The listing builds one solid part. Answer for the finished solid, in the listing's coordinates (mm). Face numbers are marked on the shaded views. A direction names the side the tool comes from. Round coordinates to 2 decimals unless told otherwise and drop trailing zeros. Write each loop counter-clockwise with the first axis right and the second up, starting at its lowest first coordinate (ties: lowest second). Pieces come first, ordered by that corner, then holes. Notation, with made-up numbers: (60.25, -40) - (118.25, -40) arc R27 cw to (118.25, -14) - close; hole circle Ø2 at (57, 41.5). An arc over 180 degrees is marked (long way). Return JSON: item names as keys, results as strings. Group by question number.
from build123d import *

# Parameters (mm, degrees)
SKETCH1_R           = 8.75
SKETCH1_R_2         = 4.05
BOSS_EXTRUDE1_DEPTH = 5
SKETCH2_W           = 5.1
SKETCH2_H           = 10
CUT_EXTRUDE3_DEPTH  = 4.1
CIRPATTERN1_COUNT   = 6


with BuildPart() as part:
    # Sketch1 → Boss-Extrude1 (new body, symmetric)
    with BuildSketch(Plane.XY):
        Circle(SKETCH1_R)
        Circle(SKETCH1_R_2, mode=Mode.SUBTRACT)
    extrude(amount=BOSS_EXTRUDE1_DEPTH, both=True)

    # Sketch2 → Cut-Extrude3 (cut)
    with BuildSketch(Plane(origin=(-8.75, -17.193061184, 0), x_dir=(0, -1, 0), z_dir=(1, 0, 0))):
        with Locations((-17.193061184, 0)):
            Rectangle(SKETCH2_W, SKETCH2_H)
    cut_extrude3 = extrude(amount=CUT_EXTRUDE3_DEPTH, mode=Mode.SUBTRACT)

    # CirPattern1: Cut-Extrude3 ×6 about axis
    cirpattern1_axis = Axis((0, 0, 0), (0, 0, 1))
    for i in range(1, CIRPATTERN1_COUNT):
        add(cut_extrude3.rotate(cirpattern1_axis, i * 360 / CIRPATTERN1_COUNT), mode=Mode.SUBTRACT)


solid = part.part
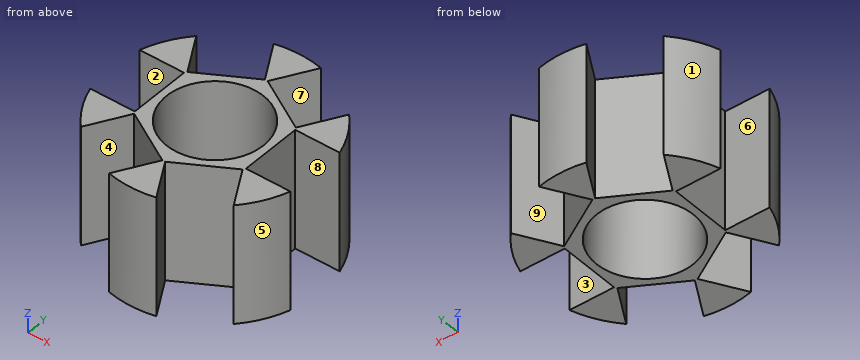
(1) Find section D-D (x = 6.75). Write down the section's boundary in (y, z), plus the area to 3 significant figures.
(2) Determine the mould class of the marked faces 1, 2, 3 and 4 for opening direction Y: +Y half, -Y half, draft (parallel to the pull), parting line (faces both ways), or undercut.
(3) Find section C-C (x = 1.75). Write down the section's boundary in (y, z), plus the area to 3 significant figures.
(4) Consider line 1 (X direction, y = -3.5, z = 1.75); line 2 (X direction, y = 3.25, z = -0.75); line 3 (X direction, y = 4.5, z = -0.75). Determine where each line is inside the solid, lowest interval first.
(5) For the marked faces 5, 6, 7, 8 and 9, determine the directions among +Z, -Z, +X, -X, +Y, -Y from which every point of the face is accessible in a straight line to the end or side of a thin tool.
(6) Find section A-A (z = -2.25). Write down the section's boundary in (x, y), plus the area to 3 significant figures.
(7) Flat-ended cylindrical pins translate along their axes: pin 1 (3 mm diameter, centred on x = -7, z = 2, fed in from +Y); pin 2 (1.5 mm diameter, centred on y = 0, z = -1.5, fed in from +X); pin 3 (1.9 mm diameter, centred on x = 6.5, z = 0, fed in from -Y). Find the tip coordinate at first contact, or state that the pin passes through.
(8) Find section B-B (y = 0). Write down the section's boundary in (x, z), plus the area to 3 significant figures.
Check sheet entries:
{
 "1": {"outline": "(-5.57, -5) - (-2.55, -5) - (-2.55, 5) - (-5.57, 5) - close; (2.55, -5) - (5.57, -5) - (5.57, 5) - (2.55, 5) - close", "area": "60.4 mm^2"},
 "2": {"face 1": "+Y half", "face 2": "undercut", "face 3": "undercut", "face 4": "-Y half"},
 "3": {"outline": "(-8.57, -5) - (-8.13, -5) - (-8.13, 5) - (-8.57, 5) - close; (-4.36, -5) - (-3.65, -5) - (-3.65, 5) - (-4.36, 5) - close; (3.65, -5) - (4.36, -5) - (4.36, 5) - (3.65, 5) - close; (8.13, -5) - (8.57, -5) - (8.57, 5) - (8.13, 5) - close", "area": "23.0 mm^2"},
 "4": {"line 1": "x = -8.02 to -4.97, -3.24 to -2.04, 2.04 to 3.24, 4.97 to 8.02", "line 2": "x = -8.12 to -4.82, -3.67 to -2.42, 2.42 to 3.67, 4.82 to 8.12", "line 3": "x = -7.5 to -5.54, -1.51 to 1.51, 5.54 to 7.5"},
 "5": {"face 5": "+Z, -Z, +X, -Y", "face 6": "+Z, -Z, -X", "face 7": "+Z, -Z", "face 8": "+Z, -Z, +X", "face 9": "+Z, -Z, +Y"},
 "6": {"outline": "(-8.37, -2.55) arc R8.75 ccw to (-6.39, -5.97) - (-4.53, -2.75) - (-0.12, -5.3) - (-1.98, -8.52) arc R8.75 ccw to (1.98, -8.52) - (0.12, -5.3) - (4.53, -2.75) - (6.39, -5.97) arc R8.75 ccw to (8.37, -2.55) - (4.65, -2.55) - (4.65, 2.55) - (8.37, 2.55) arc R8.75 ccw to (6.39, 5.97) - (4.53, 2.75) - (0.12, 5.3) - (1.98, 8.52) arc R8.75 ccw to (-1.98, 8.52) - (-0.12, 5.3) - (-4.53, 2.75) - (-6.39, 5.97) arc R8.75 ccw to (-8.37, 2.55) - (-4.65, 2.55) - (-4.65, -2.55) - close; hole circle Ø8.1 at (0, 0)", "area": "67.4 mm^2"},
 "7": {"pin 1": "stops at y = 5.97", "pin 2": "stops at x = 4.65", "pin 3": "stops at y = -5.97"},
 "8": {"outline": "(-4.65, -5) - (-4.05, -5) - (-4.05, 5) - (-4.65, 5) - close; (4.05, -5) - (4.65, -5) - (4.65, 5) - (4.05, 5) - close", "area": "12.0 mm^2"}
}
